Geometry check sheet. Reference: the model listing, model coordinates, mm. Face numbers are marked on the shaded views. A direction names the side the tool comes from. Give positions to 0.01 mm unless a question says otherwise; leave off trailing zeros. Write each loop counter-clockwise with the first axis right and the second up, starting at its lowest first coordinate (ties: lowest second). Pieces come first, ordered by that corner, then holes.
(1) Cross-section at A-A (y = 8.5). Record the boundary of the cut face in (x, z) (3 decimals).
(2) Cross-section at B-B (x = 33.5). Record the boundary of the cut face in (y, z), and give its area (3 significant figures).
(3) Cross-section at D-D (x = -14.5). Record the boundary of the cut face in (y, z), and give its area (3 significant figures).
(4) Depth check by flat-ended pin: P1, Ø5, axis at x = 32, y = 4, coming from the +Z side; P2, Ø3, axis at x = 25, y = 3.5, coming from the -Z side; P3, Ø5, axis at x = -12.5, y = 2.5, coming from the -Z side. Enter the tip coordinate at first touch or a pass-through.
(5) Thickness scan on line 1 along X through (y, z) = (3, 4); line 2 along Z through (x, y) = (-33, 6); line 3 along Y through (x, z) = (3, 2.5). Record the ranges inside material, lowest first.
(6) Mould release check, pull along X, two halves, no side actions. Record for the marked faces 1, 2 and 3: +X half, -X half, draft (parallel to the pull), parting line (faces both ways), or undercut.
(7) Tool access check on the marked faces 4, 5, 6 and 7. Record the directions out of +Z, -Z, +X, -X, +Y, -Y that give a thin tool (end or side, any length) a straight path to the whole face; none if there is none.
```python
from build123d import *

# Parameters (mm, degrees)
SKETCH1_W           = 74
SKETCH1_H           = 18
BOSS_EXTRUDE1_DEPTH = 6.3
BOSS_EXTRUDE2_DEPTH = 12
BOSS_EXTRUDE3_DEPTH = 1
SKETCH6_R           = 2.1
CUT_EXTRUDE1_DEPTH  = 42.411834057


with BuildPart() as part:
    # Sketch1 → Boss-Extrude1 (new body)
    with BuildSketch(Plane(origin=(0, 0, 0), x_dir=(1, 0, 0), z_dir=(0, 1, 0))):
        Rectangle(SKETCH1_W, SKETCH1_H)
    extrude(amount=BOSS_EXTRUDE1_DEPTH)

    # Sketch4 → Boss-Extrude2 (add)
    with BuildSketch(Plane(origin=(0, 0, 0), x_dir=(1, 0, 0), z_dir=(0, 1, 0))):
        with BuildLine():
            Line((-27.625, 11.875), (-27.625, -11.875))
            ThreePointArc((-27.625, -11.875), (-28.5, -12.75), (-29.375, -11.875))
            Line((-29.375, -11.875), (-29.375, 11.875))
            ThreePointArc((-29.375, 11.875), (-28.5, 12.75), (-27.625, 11.875))
        make_face()
        with BuildLine():
            Line((-18.125, 11.875), (-18.125, -11.875))
            ThreePointArc((-18.125, -11.875), (-19, -12.75), (-19.875, -11.875))
            Line((-19.875, -11.875), (-19.875, 11.875))
            ThreePointArc((-19.875, 11.875), (-19, 12.75), (-18.125, 11.875))
        make_face()
        with BuildLine():
            Line((-8.625, 11.875), (-8.625, -11.875))
            ThreePointArc((-8.625, -11.875), (-9.5, -12.75), (-10.375, -11.875))
            Line((-10.375, -11.875), (-10.375, 11.875))
            ThreePointArc((-10.375, 11.875), (-9.5, 12.75), (-8.625, 11.875))
        make_face()
        with BuildLine():
            Line((0.875, 11.875), (0.875, -11.875))
            ThreePointArc((0.875, -11.875), (0, -12.75), (-0.875, -11.875))
            Line((-0.875, -11.875), (-0.875, 11.875))
            ThreePointArc((-0.875, 11.875), (0, 12.75), (0.875, 11.875))
        make_face()
        with BuildLine():
            Line((10.375, 11.875), (10.375, -11.875))
            ThreePointArc((10.375, -11.875), (9.5, -12.75), (8.625, -11.875))
            Line((8.625, -11.875), (8.625, 11.875))
            ThreePointArc((8.625, 11.875), (9.5, 12.75), (10.375, 11.875))
        make_face()
        with BuildLine():
            Line((19.875, 11.875), (19.875, -11.875))
            ThreePointArc((19.875, -11.875), (19, -12.75), (18.125, -11.875))
            Line((18.125, -11.875), (18.125, 11.875))
            ThreePointArc((18.125, 11.875), (19, 12.75), (19.875, 11.875))
        make_face()
        with BuildLine():
            Line((29.375, 11.875), (29.375, -11.875))
            ThreePointArc((29.375, -11.875), (28.5, -12.75), (27.625, -11.875))
            Line((27.625, -11.875), (27.625, 11.875))
            ThreePointArc((27.625, 11.875), (28.5, 12.75), (29.375, 11.875))
        make_face()
    extrude(amount=BOSS_EXTRUDE2_DEPTH)

    # Sketch5 → Boss-Extrude3 (add)
    with BuildSketch(Plane(origin=(0, 6.3, 0), x_dir=(1, 0, 0), z_dir=(0, 1, 0))):
        Polygon((-27.625, 11), (-26.25, 11), (-26.25, 17.5), (-21.25, 17.5), (-21.25, 11), (-19.875, 11), (-19.875, -11), (-21.25, -11), (-21.25, -17.5), (-26.25, -17.5), (-26.25, -11), (-27.625, -11), align=None)
        Polygon((-18.125, 11), (-16.75, 11), (-16.75, 17.5), (-11.75, 17.5), (-11.75, 11), (-10.375, 11), (-10.375, -11), (-11.75, -11), (-11.75, -17.5), (-16.75, -17.5), (-16.75, -11), (-18.125, -11), align=None)
        Polygon((-8.625, 11), (-7.25, 11), (-7.25, 17.5), (-2.25, 17.5), (-2.25, 11), (-0.875, 11), (-0.875, -11), (-2.25, -11), (-2.25, -17.5), (-7.25, -17.5), (-7.25, -11), (-8.625, -11), align=None)
        Polygon((0.875, 11), (2.25, 11), (2.25, 17.5), (7.25, 17.5), (7.25, 11), (8.625, 11), (8.625, -11), (7.25, -11), (7.25, -17.5), (2.25, -17.5), (2.25, -11), (0.875, -11), align=None)
        Polygon((10.375, 11), (11.75, 11), (11.75, 17.5), (16.75, 17.5), (16.75, 11), (18.125, 11), (18.125, -11), (16.75, -11), (16.75, -17.5), (11.75, -17.5), (11.75, -11), (10.375, -11), align=None)
        Polygon((19.875, 11), (21.25, 11), (21.25, 17.5), (26.25, 17.5), (26.25, 11), (27.625, 11), (27.625, -11), (26.25, -11), (26.25, -17.5), (21.25, -17.5), (21.25, -11), (19.875, -11), align=None)
    extrude(amount=BOSS_EXTRUDE3_DEPTH)

    # Sketch6 → Cut-Extrude1 (cut, through all)
    with BuildSketch(Plane(origin=(0, 6.3, 0), x_dir=(1, 0, 0), z_dir=(0, 1, 0))):
        with Locations(Location((-33.5, 4, 0), (0, 0, 270))):
            Circle(SKETCH6_R)
        with Locations(Location((-33.5, -4, 0), (0, 0, 270))):
            Circle(SKETCH6_R)
        with Locations(Location((33.5, 4, 0), (0, 0, 270))):
            Circle(SKETCH6_R)
        with Locations(Location((33.5, -4, 0), (0, 0, 270))):
            Circle(SKETCH6_R)
    extrude(amount=-CUT_EXTRUDE1_DEPTH, mode=Mode.SUBTRACT)


solid = part.part
```
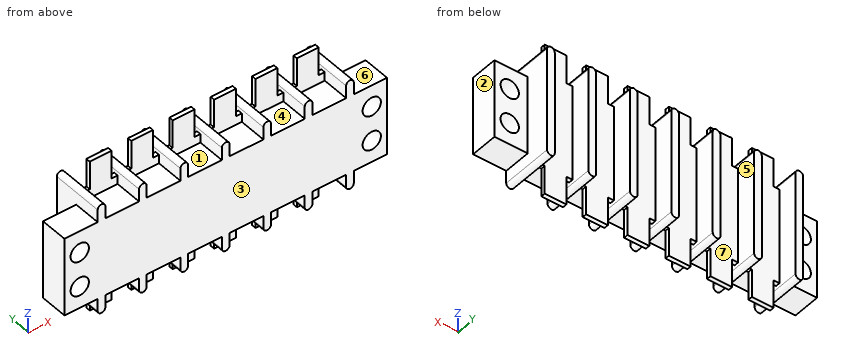
Reply:
1. outline: (-29.375, -11.875) arc R0.875 ccw to (-27.625, -11.875) - (-27.625, 11.875) arc R0.875 ccw to (-29.375, 11.875) - close; (-19.875, -11.875) arc R0.875 ccw to (-18.125, -11.875) - (-18.125, 11.875) arc R0.875 ccw to (-19.875, 11.875) - close; (-10.375, -11.875) arc R0.875 ccw to (-8.625, -11.875) - (-8.625, 11.875) arc R0.875 ccw to (-10.375, 11.875) - close; (-0.875, -11.875) arc R0.875 ccw to (0.875, -11.875) - (0.875, 11.875) arc R0.875 ccw to (-0.875, 11.875) - close; (8.625, -11.875) arc R0.875 ccw to (10.375, -11.875) - (10.375, 11.875) arc R0.875 ccw to (8.625, 11.875) - close; (18.125, -11.875) arc R0.875 ccw to (19.875, -11.875) - (19.875, 11.875) arc R0.875 ccw to (18.125, 11.875) - close; (27.625, -11.875) arc R0.875 ccw to (29.375, -11.875) - (29.375, 11.875) arc R0.875 ccw to (27.625, 11.875) - close
2. outline: (0, -9) - (6.3, -9) - (6.3, -6.1) - (0, -6.1) - close; (0, -1.9) - (6.3, -1.9) - (6.3, 1.9) - (0, 1.9) - close; (0, 6.1) - (6.3, 6.1) - (6.3, 9) - (0, 9) - close
2. area: 60.5 mm2
3. outline: (0, -9) - (6.3, -9) - (6.3, -17.5) - (7.3, -17.5) - (7.3, 17.5) - (6.3, 17.5) - (6.3, 9) - (0, 9) - close
3. area: 148 mm2
4. P1: stops at z = 9
4. P2: stops at z = -9
4. P3: stops at z = -12.59
5. line 1: x = -37 to -35.6, -31.4 to 31.4, 35.6 to 37
5. line 2: z = -9 to -6.04, -1.96 to 1.96, 6.04 to 9
5. line 3: y = 0 to 7.3
6. face 1: undercut
6. face 2: +X half
6. face 3: draft
7. face 4: +Z, -Y
7. face 5: none
7. face 6: +Z, +X, +Y, -Y
7. face 7: +Z, -Z, +Y
